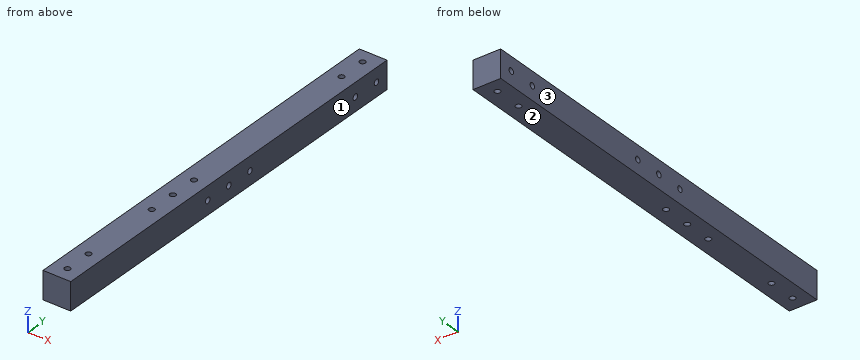
from build123d import *

# Parameters (mm, degrees)
SKETCH_1_W          = 20
SKETCH_1_H          = 20
EXTRUDE_1_DEPTH     = 300
SKETCH_2_R          = 2.1
CUT_EXTRUDE_1_DEPTH = 301.83217913
SKETCH_4_R          = 2.1
CUT_EXTRUDE_2_DEPTH = 301.83217913
SKETCH_5_R          = 2.1
CUT_EXTRUDE_3_DEPTH = 301.83217913
SKETCH_6_R          = 2.1
CUT_EXTRUDE_4_DEPTH = 301.83217913


with BuildPart() as part:
    # 草图1 → 凸台-拉伸1 (new body)
    with BuildSketch(Plane(origin=(0, 0, 0), x_dir=(1, 0, 0), z_dir=(0, 1, 0))):
        Rectangle(SKETCH_1_W, SKETCH_1_H)
    extrude(amount=EXTRUDE_1_DEPTH)

    # 草图2 → 切除-拉伸1 (cut, through all)
    with BuildSketch(Plane.XY.offset(10)):
        with Locations((0, 10)):
            Circle(SKETCH_2_R)
        with Locations((0, 30)):
            Circle(SKETCH_2_R)
        with Locations(Location((0, 270, 0), (0, 0, 180))):
            Circle(SKETCH_2_R)
        with Locations(Location((0, 290, 0), (0, 0, 180))):
            Circle(SKETCH_2_R)
    extrude(amount=-CUT_EXTRUDE_1_DEPTH, mode=Mode.SUBTRACT)

    # 草图4 → 切除-拉伸2 (cut, through all)
    with BuildSketch(Plane.ZY.offset(10)):
        with Locations((0, 130)):
            Circle(SKETCH_4_R)
        with Locations((0, 150)):
            Circle(SKETCH_4_R)
        with Locations((0, 170)):
            Circle(SKETCH_4_R)
    extrude(amount=-CUT_EXTRUDE_2_DEPTH, mode=Mode.SUBTRACT)

    # 草图5 → 切除-拉伸3 (cut, through all)
    with BuildSketch(Plane(origin=(10, 0, 0), x_dir=(0, 0, -1), z_dir=(1, 0, 0))):
        with Locations((0, 290)):
            Circle(SKETCH_5_R)
        with Locations((0, 270)):
            Circle(SKETCH_5_R)
    extrude(amount=-CUT_EXTRUDE_3_DEPTH, mode=Mode.SUBTRACT)

    # 草图6 → 切除-拉伸4 (cut, through all)
    with BuildSketch(Plane(origin=(0, 0, -10), x_dir=(-1, 0, 0), z_dir=(0, 0, -1))):
        with Locations((0, 90)):
            Circle(SKETCH_6_R)
        with Locations((0, 110)):
            Circle(SKETCH_6_R)
        with Locations((0, 130)):
            Circle(SKETCH_6_R)
    extrude(amount=-CUT_EXTRUDE_4_DEPTH, mode=Mode.SUBTRACT)


solid = part.part
The model under review builds one solid part; all positions refer to its coordinate system, in mm. Face numbers are marked on the shaded views. Coordinates: 2 decimals unless noted, no trailing zeros. Write each loop counter-clockwise with the first axis right and the second up, starting at its lowest first coordinate (ties: lowest second). Pieces come first, ordered by that corner, then holes. Notation, with made-up numbers: (18, -6) -> (33, -6) arc R24 ccw to (33, 32) -> close; hole circle Ø3 at (48, 71). An arc over 180 degrees is marked (long way). Answer in a Markdown table with one row per item.
1. Wall thickness on probe 1 along Y at (x, z) = (-2.75, 0); probe 2 along X at (y, z) = (290, -7); probe 3 along Y at (x, z) = (2.25, 1.75): over which ranges is each line inside the solid? List them lowest first. Write a range as [from, to].
Answers below:
| item | result |
|---|---|
| probe 1 | y = [0, 127.9], [132.1, 147.9], [152.1, 167.9], [172.1, 267.9], [272.1, 287.9], [292.1, 300] |
| probe 2 | x = [-10, -2.1], [2.1, 10] |
| probe 3 | y = [0, 128.84], [131.16, 148.84], [151.16, 168.84], [171.16, 268.84], [271.16, 288.84], [291.16, 300] |
2. We need section A-A, the plane z = -5. State the section outline as (x, y) points, and give its area (3 significant figures).
Answers below:
| item | result |
|---|---|
| outline | (-10, 0) -> (10, 0) -> (10, 300) -> (-10, 300) -> close; hole circle Ø4.2 at (0, 10); hole circle Ø4.2 at (0, 30); hole circle Ø4.2 at (0, 90); hole circle Ø4.2 at (0, 110); hole circle Ø4.2 at (0, 130); hole circle Ø4.2 at (0, 270); hole circle Ø4.2 at (0, 290) |
| area | 5,900 mm^2 |
3. Draft analysis for pull direction X (two halves, no side actions). For the marked faces 1, 2 and 3, state which applies: +X half, -X half, draft (parallel to the pull), parting line (faces both ways), or undercut.
Answers below:
| item | result |
|---|---|
| face 1 | +X half |
| face 2 | draft |
| face 3 | -X half |
4. Clearance check with a flat-ended pin moving along its axis: pin 1 Ø4 at (x, y) = (0, 270) entering from -Z. State where the tip first meets the part, or that it passes through.
Answers below:
| item | result |
|---|---|
| pin 1 | passes through |
